```python
from build123d import *

# Parameters (mm, degrees)
F0_W      = 31.75
F0_H      = 43.942
F1_DEPTH  = 8.509
F3_DEPTH  = 25.4
F4_R      = 0.889
F5_DEPTH  = 31.75
F7_DEPTH  = 9.525
F9_DEPTH  = 3.429
F10_DEPTH = 6.35
F11_W     = 6.35
F11_H     = 43.942
F12_DEPTH = 60.325
F13_W     = 6.35
F13_H     = 10.16
F14_DEPTH = 6.35
F16_DEPTH = 43.942
F17_DEPTH = 25.4
F19_DEPTH = 9.525
F20_R     = 3.175
F21_R     = 3.175
F22_R     = 0.889
F23_DEPTH = 7.62


with BuildPart() as f1:
    # F0 (on Right) → F1 (new body)
    with BuildSketch(Plane.YZ):
        with Locations((15.875, -21.971)):
            Rectangle(F0_W, F0_H)
    extrude(amount=F1_DEPTH)

    # F2 (on face) → F3 (cut)
    with BuildSketch(Plane(origin=(0, 0, 0), x_dir=(0, -1, 0), z_dir=(-1, 0, 0))):
        Polygon((0, 0), (-9.525, 0), (0, -1.3335), align=None)
        Polygon((0, -43.942), (0, -42.6085), (-9.525, -43.942), align=None)
    extrude(amount=-F3_DEPTH, mode=Mode.SUBTRACT)

    # F4 (on face) → F5 (cut)
    with BuildSketch(Plane(origin=(0, 31.75, 0), x_dir=(-1, 0, 0), z_dir=(0, 1, 0))):
        with Locations((-4.2545, -37.846)):
            Circle(F4_R)
        with Locations((-4.2545, -6.096)):
            Circle(F4_R)
    extrude(amount=-F5_DEPTH, mode=Mode.SUBTRACT)

    # F6 (on face) → F7 (cut)
    with BuildSketch(Plane.XZ):
        with BuildLine():
            Line((0, -37.846), (3.3655, -37.846))
            ThreePointArc((3.3655, -37.846), (4.2545, -36.957), (5.1435, -37.846))
            Line((5.1435, -37.846), (6.2865, -37.846))
            Line((6.2865, -37.846), (6.2865, -21.971))
            Line((6.2865, -21.971), (6.2865, -6.096))
            Line((6.2865, -6.096), (5.1435, -6.096))
            ThreePointArc((5.1435, -6.096), (4.2545, -6.985), (3.3655, -6.096))
            Line((3.3655, -6.096), (0, -6.096))
            Line((0, -6.096), (0, -37.846))
        make_face()
    extrude(amount=-F7_DEPTH, mode=Mode.SUBTRACT)

    # F8 (on face) → F9 (join)
    with BuildSketch(Plane(origin=(0, 0, 0), x_dir=(0, -1, 0), z_dir=(-1, 0, 0))):
        Polygon((-9.525, -37.846), (-9.525, -6.096), (-9.525, 0), (-31.75, 0), (-31.75, -43.942), (-9.525, -43.942), align=None)
    extrude(amount=F9_DEPTH)

    # F10 (add): a face of the model
    f10_faces = [f1.faces().sort_by_distance(p)[0] for p in [
        (-3.429, 20.6375, -21.971),
    ]]
    extrude(f10_faces, amount=F10_DEPTH)

    # F11 (on face) → F12 (join)
    with BuildSketch(Plane.XZ.offset(-9.525)):
        with Locations((-6.604, -21.971)):
            Rectangle(F11_W, F11_H)
    extrude(amount=F12_DEPTH)

    # F13 (on face) → F14 (cut)
    with BuildSketch(Plane.YZ.offset(-3.429)):
        with Locations((-42.418, -27.051)):
            Rectangle(F13_W, F13_H)
        with Locations((-42.418, -16.891)):
            Rectangle(F13_W, F13_H)
    extrude(amount=-F14_DEPTH, mode=Mode.SUBTRACT)

    # F15 (on face) → F16 (join, through all)
    with BuildSketch(Plane.XY):
        Polygon((-3.429, -20.6375), (-3.429, -50.8), (-1.8415, -50.8), align=None)
    extrude(amount=-F16_DEPTH)

    # F17 (cut): a face of the model
    f17_faces = [f1.faces().sort_by_distance(p)[0] for p in [
        (-3.429, -42.418, -21.971),
    ]]
    extrude(f17_faces, amount=-F17_DEPTH, mode=Mode.SUBTRACT)

    # F18 (on face) → F19 (cut)
    with BuildSketch(Plane(origin=(-9.779, 0, 0), x_dir=(0, -1, 0), z_dir=(-1, 0, 0))):
        Polygon((-9.525, 0), (50.8, -6.4365183935), (50.8, 0), align=None)
        Polygon((50.8, -43.942), (50.8, -38.0690358579), (-9.525, -43.942), align=None)
    extrude(amount=-F19_DEPTH, mode=Mode.SUBTRACT)

    # F20
    f20_edges = [f1.edges().sort_by_distance(p)[0] for p in [
        (-1.8415, -50.8, -22.252777),
    ]]
    fillet(f20_edges, radius=F20_R)

    # F21
    f21_edges = [f1.edges().sort_by_distance(p)[0] for p in [
        (-9.779, -50.8, -22.252777),
    ]]
    fillet(f21_edges, radius=F21_R)

    # F22 (on face) → F23 (cut)
    with BuildSketch(Plane(origin=(0, 31.75, 0), x_dir=(-1, 0, 0), z_dir=(0, 1, 0))):
        with BuildLine():
            ThreePointArc((-6.7945, -6.096), (-4.2545, -8.636), (-1.7145, -6.096))
            ThreePointArc((-1.7145, -6.096), (-4.2545, -3.556), (-6.7945, -6.096))
        make_face()
        with Locations((-4.2545, -6.096)):
            Circle(F22_R, mode=Mode.SUBTRACT)
        with BuildLine():
            Line((-1.7145, -37.846), (-1.7145, -6.096))
            ThreePointArc((-1.7145, -6.096), (-4.2545, -8.636), (-6.7945, -6.096))
            Line((-6.7945, -6.096), (-6.7945, -37.846))
            ThreePointArc((-6.7945, -37.846), (-4.2545, -35.306), (-1.7145, -37.846))
        make_face()
        with BuildLine():
            ThreePointArc((-6.7945, -37.846), (-4.2545, -40.386), (-1.7145, -37.846))
            ThreePointArc((-1.7145, -37.846), (-4.2545, -35.306), (-6.7945, -37.846))
        make_face()
        with Locations((-4.2545, -37.846)):
            Circle(F22_R, mode=Mode.SUBTRACT)
    extrude(amount=-F23_DEPTH, mode=Mode.SUBTRACT)


solid = f1.part
```
Part model, mm, in its own coordinate system. A direction names the side the tool comes from. Coordinates: 2 decimals unless noted, no trailing zeros. Write each loop counter-clockwise with the first axis right and the second up, starting at its lowest first coordinate (ties: lowest second). Pieces come first, ordered by that corner, then holes.
Item 1: Pin check, flat tips, straight feed: pin 1 (5 mm diameter, centred on x = 2.5, z = -25.5, fed in from -Y) (3 decimals); pin 2 (2 mm diameter, centred on x = 3.5, z = -5.5, fed in from +Y); pin 3 (0.6 mm diameter, centred on x = 5.5, y = 2.5, fed in from -Z); pin 4 (1.4 mm diameter, centred on x = 4.25, z = -6.1, fed in from +Y). Stop position of each tip, or through.
Item 2: Probe line 1 (X direction, y = 5.5, z = -18); line 2 (Y direction, x = -6.5, z = -12); line 3 (Y direction, x = -3.75, z = -26). List the from-to ranges inside material, lowest first.
Item 3: Slice it at D-D (y = -19). Write the cut outline in (x, z), and give its area (3 significant figures).
Item 4: Which spindle directions (+Z, -Z, +X, -X, +Y, -Y) get a long thin tool onto all of the face, cutting with end or side? Do faces 5 (the face through (-2.87, -31.26, -21.85)), 6 (the face through (4, 24.13, -22)), 7 (the face through (-6, -45.593, -22)), 8 (the face through (-3.429, -5, -22)). Say none if no direction does.
Item 5: Mould opens along Z. For faces 1 (the face through (-1, 21, 0)), 2 (the face through (0, 5, -41)), 3 (the face through (4.195, 4.696, -43.266)), 4 (the face through (4.199, 27.993, -3.557)) say: released by +Z, released by -Z, zero draft, split by the parting line, or undercut.
Item 6: Slice it at B-B (y = 8). Write the cut outline in (x, z), and give its area (3 significant figures).
Results found:
1. pin 1: stops at y = 9.525
1. pin 2: stops at y = 24.13
1. pin 3: stops at z = -43
1. pin 4: passes through
2. line 1: x = -9.78 to -3.43, 6.29 to 8.51
2. line 2: y = -50.8 to -45.59, -39.24 to 31.75
2. line 3: y = -50.46 to -45.59, -39.24 to 31.75
3. outline: (-9.78, -41.16) - (-3.43, -41.16) - (-3.43, -3.04) - (-9.78, -3.04) - close
3. area: 242 mm2
4. face 5: +Z, -Z, +X
4. face 6: +Y
4. face 7: +X, -X
4. face 8: +Z, -Z
5. face 1: released by +Z
5. face 2: zero draft
5. face 3: released by -Z
5. face 4: undercut
6. outline: (-9.78, -43.79) - (-3.43, -43.79) - (-3.43, -0.16) - (-9.78, -0.16) - close; (0, -43.73) - (8.51, -43.73) - (8.51, -0.21) - (0, -0.21) - (0, -6.1) - (3.37, -6.1) arc R0.89 cw to (5.14, -6.1) - (6.29, -6.1) - (6.29, -37.85) - (5.14, -37.85) arc R0.89 cw to (3.37, -37.85) - (0, -37.85) - close
6. area: 445 mm2
